Build history of the part. All positions in model axes, mm. Face numbers are marked on the shaded views. Give positions to 0.01 mm unless a question says otherwise; leave off trailing zeros. Write each loop counter-clockwise with the first axis right and the second up, starting at its lowest first coordinate (ties: lowest second). Pieces come first, ordered by that corner, then holes. Notation, with made-up numbers: (32.25, 41.25) -> (81.25, 41.25) arc R22 ccw to (81.25, 53.25) -> close; hole circle Ø7 at (14.25, -30.5). An arc over 180 degrees is marked (long way). Put each result on its own line as item: value.
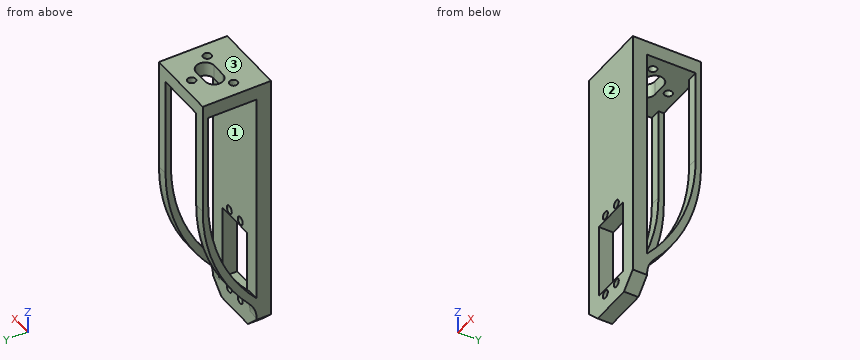
Autodesk Inventor part; units mm, degrees
ref_plane "YZ Plane" through (0, 0, 0) normal (1, 0, 0) x (0, 1, 0)
ref_plane "XZ Plane" through (0, 0, 0) normal (0, 1, 0) x (-1, 0, 0)
ref_plane "XY Plane" through (0, 0, 0) normal (0, 0, 1) x (1, 0, 0)
sketch "Sketch1" plane through (0, 0, 0) normal (1, 0, 0) x (0, 1, 0)
  line L0 (0, 0) -> (8, 0)
  line L1 (8, 0) -> (8, 150)
  line L2 (8, 150) -> (0, 150)
  line L3 (0, 150) -> (0, 0)
  dimension "d0" = 150
  dimension "d1" = 8
extrude "BODY1" add sketch "Sketch1" against normal blind 40
sketch "Sketch2" plane through (0, 8, 150) normal (0, 1, 0) x (1, 0, 0)
  line L0 (0, 0) -> (-40, 0)
  line L1 (-40, 0) -> (-40, 8)
  line L2 (-40, 8) -> (0, 8)
  line L3 (0, 8) -> (0, 0)
  dimension "d4" = 40
  dimension "d5" = 8
extrude "BODY2" add sketch "Sketch2" along normal blind 30
sketch "Sketch3" plane through (-40, 8, 0) normal (0, 1, 0) x (1, 0, 0)
  line L0 (40, 0) -> (0, 0) construction
  line L1 (0, -142) -> (0, 0) construction
  circle A0 centre (15, -10) radius 2.25
  circle A1 centre (25, -10) radius 2.25
  circle A2 centre (15, -58) radius 2.25
  circle A3 centre (25, -58) radius 2.25
  line L2 (9, -13) -> (31, -13)
  line L3 (31, -13) -> (31, -55)
  line L4 (31, -55) -> (9, -55)
  line L5 (9, -55) -> (9, -13)
  dimension "d8" = 48
  dimension "d9" = 48
  dimension "d10" = 10
  dimension "d11" = 10
  dimension "d12" = 4.5
  dimension "d13" = 4.5
  dimension "d14" = 4.5
  dimension "d15" = 4.5
  dimension "d16" = 15
  dimension "d17" = 10
  dimension "d18" = 15
  dimension "d19" = 10
  dimension "d20" = 22
  dimension "d21" = 42
  dimension "d22" = 9
  dimension "d23" = 3
extrude "SERVO" cut sketch "Sketch3" against normal blind 8
sketch "Sketch4" plane through (0, 8, 142) normal (0, 0, -1) x (-1, 0, 0)
  line L0 (40, 0) -> (0, 0) construction
  line L1 (40, 0) -> (40, 30) construction
  line L2 (0, 30) -> (40, 30) construction
  line L3 (0, 0) -> (0, 30) construction
  line L4 (24, 19) -> (16, 19)
  line L5 (16, 19) -> (16, 9)
  line L6 (16, 9) -> (24, 9)
  line L7 (24, 9) -> (24, 19)
  arc A0 (24, 9) -> (24, 19) centre (24, 14) ccw
  arc A1 (16, 19) -> (16, 9) centre (16, 14) ccw
  circle A2 centre (20, 24) radius 2.25
  circle A3 centre (32, 8) radius 2.25
  circle A4 centre (8, 8) radius 2.25
  point P0 (0, -8)
  dimension "d26" = 11
  dimension "d28" = 8
  dimension "d29" = 10
  dimension "d30" = 16
  dimension "d32" = 4.5
  dimension "d33" = 4.5
  dimension "d34" = 4.5
  dimension "d35" = 20
  dimension "d36" = 8
  dimension "d37" = 8
  dimension "d39" = 6
  dimension "d40" = 8
  dimension "d41" = 8
extrude "CONNECTION" cut sketch "Sketch4" against normal blind 8
chamfer "v3_servo_chamfer" distance 8 angle 45 2 edges at (0, 4, 0) (-40, 4, 0)
sketch "v3_ribs_sketch" plane through (0, 8, 142) normal (0, 0, -1) x (-1, 0, 0)
  line L0 (0, 30) -> (0, -8) construction
  line L1 (0, 30) -> (6, 30)
  line L2 (6, 30) -> (6, 27)
  line L3 (6, 27) -> (0, 27)
  line L4 (0, 27) -> (0, 30)
  line L5 (40, 30) -> (0, 30) construction
  line L6 (40, 30) -> (34, 30)
  line L7 (34, 30) -> (34, 27)
  line L8 (34, 27) -> (40, 27)
  line L9 (40, 27) -> (40, 30)
  dimension "d66" = 6
  dimension "d67" = 3
  dimension "d68" = 6
  dimension "d69" = 3
sketch "Sketch8" plane through (-40, 8, 142) normal (0, 1, 0) x (1, 0, 0)
  line L0 (0, 0) -> (0, 134) construction
  line L1 (40, 134) -> (40, 0) construction
  line L2 (32, 142) -> (8, 142) construction
  line L3 (40, 127) -> (34, 127)
  line L4 (34, 127) -> (34, 121)
  line L5 (34, 121) -> (40, 121)
  line L6 (40, 121) -> (40, 127)
  line L7 (0, 127) -> (6, 127)
  line L8 (6, 127) -> (6, 121)
  line L9 (6, 121) -> (0, 121)
  line L10 (0, 121) -> (0, 127)
  point P0 (40, 142)
  dimension "d70" = 6
  dimension "d71" = 6
  dimension "d72" = 6
  dimension "d73" = 6
  dimension "d74" = 15
  dimension "d75" = 15
extrude "v3_ribs_extrusion1" add sketch "Sketch8" along normal blind 30
extrude "v3_ribs_extrusion2" add sketch "v3_ribs_sketch" along normal blind 122
chamfer "v3_ribs_chamfer1" distance 27 angle 45 2 edges at (-3, 35, 21) (-37, 35, 21)
fillet "v3_ribs_fillet1" radius 100 2 edges at (-3, 35, 47.9999) (-37, 35, 47.9999)
fillet "v3_ribs_fillet2" radius 100 2 edges at (-3, 38, 15) (-37, 38, 15)
fillet "v3_ribs_fillet3" radius 15 2 edges at (-3, 8, 15) (-37, 8, 15)
equation "\"d4\" = d2"
equation "\"d5\" = d1"
equation "\"d9\" = d8"
equation "\"d11\" = d10"
equation "\"d13\" = d12"
equation "\"d14\" = d12"
equation "\"d15\" = d12"
equation "\"d18\" = d16"
equation "\"d19\" = d17"
equation "\"d32\" = d12"
equation "\"d33\" = d12"
equation "\"d34\" = d12"
equation "\"d37\" = d36"
equation "\"d41\" = d40"
equation "\"d68\" = d66"
equation "\"d69\" = d67"
equation "\"d70\" = d72"
equation "\"d71\" = d72"
equation "\"d72\" = d66"
equation "\"d73\" = d66"
equation "\"d75\" = d74"
properties part number "BONE_v3" material "PLA plastic"
1) Wall check: L1, parallel to X at y = 5.5, z = 58; L2, parallel to Z at x = -25, y = 3; L3, parallel to Y at x = -20, z = 145. Give the ranges that are in metal, low to high.
Filled sheet:
L1: -40 to -27.25, -22.75 to -17.25, -12.75 to 0
L2: 0 to 7.75, 12.25 to 13, 55 to 55.75, 60.25 to 150
L3: 0 to 17, 27 to 29.75, 34.25 to 38
2) Slice it at A-A (x = -20). Write the cut outline in (y, z).
Filled sheet:
outline: (0, 0) -> (8, 0) -> (8, 13) -> (0, 13) -> close; (0, 55) -> (8, 55) -> (8, 142) -> (17, 142) -> (17, 150) -> (0, 150) -> close; (27, 142) -> (29.75, 142) -> (29.75, 150) -> (27, 150) -> close; (34.25, 142) -> (38, 142) -> (38, 150) -> (34.25, 150) -> close
3) Pin check, flat tips, straight feed: pin 1 (9 mm diameter, centred on x = -19, y = 27, fed in from -Z); pin 2 (5 mm diameter, centred on y = 11.5, z = 59, fed in from +X); pin 3 (5 mm diameter, centred on x = -29.5, z = 97, fed in from +Y); pin 4 (5 mm diameter, centred on x = -32, y = 16, fed in from -Z). Stop position of each tip, or through.
Filled sheet:
pin 1: z = 142
pin 2: through
pin 3: y = 8
pin 4: z = 22.01
4) Slice it at B-B (z = 111). Write the cut outline in (x, y), plus the area to 3 significant figures.
Filled sheet:
outline: (-40, 0) -> (0, 0) -> (0, 8) -> (-40, 8) -> close; (-40, 35) -> (-34, 35) -> (-34, 38) -> (-40, 38) -> close; (-6, 35) -> (0, 35) -> (0, 38) -> (-6, 38) -> close
area: 356 mm2
5) Slice it at D-D (y = 32). Write the cut outline in (x, z), plus the area to 3 significant figures.
Filled sheet:
outline: (-40, 52.3) -> (-34, 52.3) -> (-34, 65.03) -> (-40, 65.03) -> close; (-40, 142) -> (-22.25, 142) -> (-22.25, 150) -> (-40, 150) -> close; (-17.75, 142) -> (0, 142) -> (0, 150) -> (-17.75, 150) -> close; (-6, 52.3) -> (0, 52.3) -> (0, 65.03) -> (-6, 65.03) -> close
area: 437 mm2
6) Pull direction Z, two halves, no side cores. Call the marked faces 1, 2 and 3: released by +Z, released by -Z, zero draft, split by the parting line, or undercut.
Filled sheet:
face 1: undercut
face 2: zero draft
face 3: released by +Z
